Print and shaded views of the part. All mm, measured from the part's lowest x, y and z. A direction names the side the tool comes from. Round coordinates to 2 decimals unless told otherwise and drop trailing zeros. Order: outer loops, then holes, each group sorted by start corner. A loop starts at its lowest first (then second) coordinate and runs counter-clockwise, first axis right, second up.
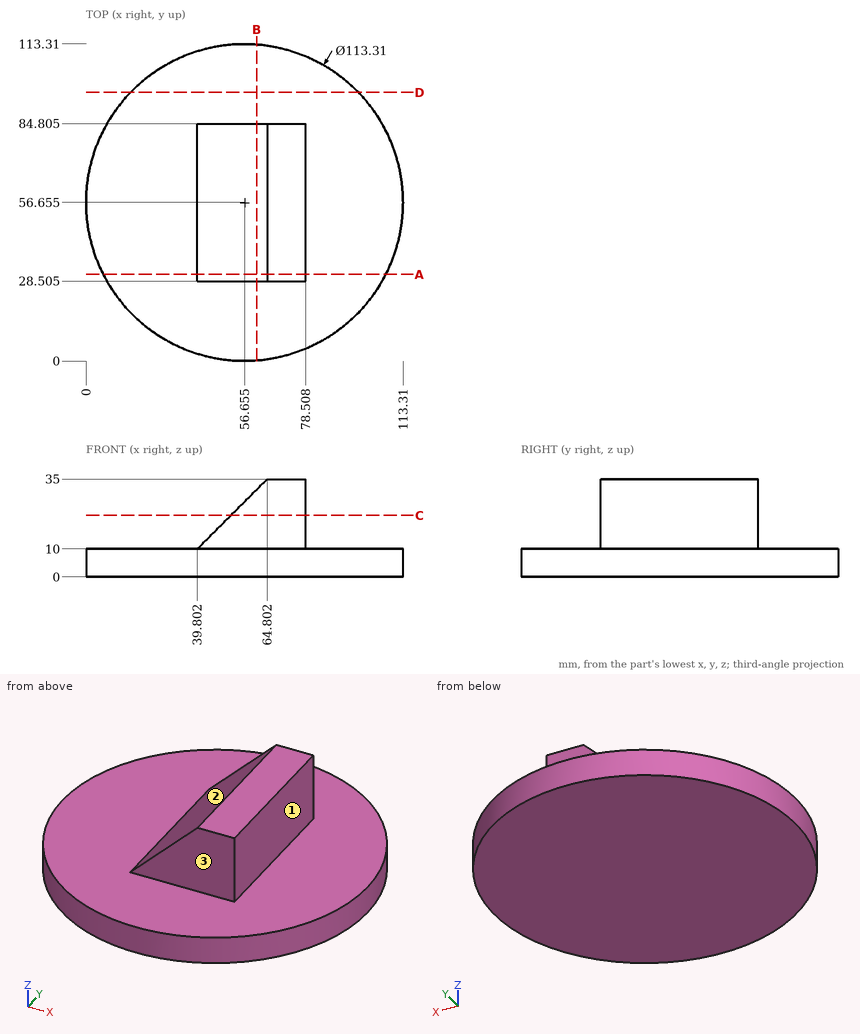
1. Drill centre lines: line 1 (Z direction, x = 103, y = 72); line 2 (Y direction, x = 77.5, z = 30) (1 decimal); line 3 (Z direction, x = 57, y = 75.5). Where is each one in solid material? Low to high.
2. Tool access for the marked faces 1, 2 and 3: list every direction of +Z, -Z, +X, -X, +Y, -Y with a clear straight run to the whole face (end or side of a thin tool).
3. Cut at C-C, the plane z = 22. Write the cut outline in (x, y) (1 decimal), and give its area (3 significant figures).
4. Cut at D-D, the plane y = 96. Write the cut outline in (x, z), and give its area (3 significant figures).
5. Pin check, flat tips, straight feed: P1, Ø5, axis at x = 80.5, z = 20.5, coming from the +Y side (3 decimals); P2, Ø12, axis at y = 42, z = 29.5, coming from the +X side; P3, Ø4, axis at x = 47, z = 6, coming from the +Y side; P4, Ø1.5, axis at y = 27, z = 28, coming from the +X side. Stop position of each tip, or through.
6. Cut at B-B, the plane x = 61. Write the cut outline in (y, z) (1 decimal).
7. Cut at A-A, the plane y = 31. Write the cut outline in (x, z), and give its area (3 significant figures).
Outcome:
1. line 1: z = 0 to 10
1. line 2: y = 28.5 to 84.8
1. line 3: z = 0 to 27.2
2. face 1: +Z, +X, +Y, -Y
2. face 2: +Z, -X, +Y, -Y
2. face 3: +Z, +X, -X, -Y
3. outline: (51.8, 28.5) - (78.5, 28.5) - (78.5, 84.8) - (51.8, 84.8) - close
3. area: 1,500 mm2
4. outline: (15.89, 0) - (97.42, 0) - (97.42, 10) - (15.89, 10) - close
4. area: 815 mm2
5. P1: stops at y = 84.805
5. P2: stops at x = 78.51
5. P3: stops at y = 112.79
5. P4: passes through
6. outline: (0.2, 0) - (113.1, 0) - (113.1, 10) - (84.8, 10) - (84.8, 31.2) - (28.5, 31.2) - (28.5, 10) - (0.2, 10) - close
7. outline: (6.14, 0) - (107.17, 0) - (107.17, 10) - (78.51, 10) - (78.51, 35) - (64.8, 35) - (39.8, 10) - (6.14, 10) - close
7. area: 1,670 mm2
